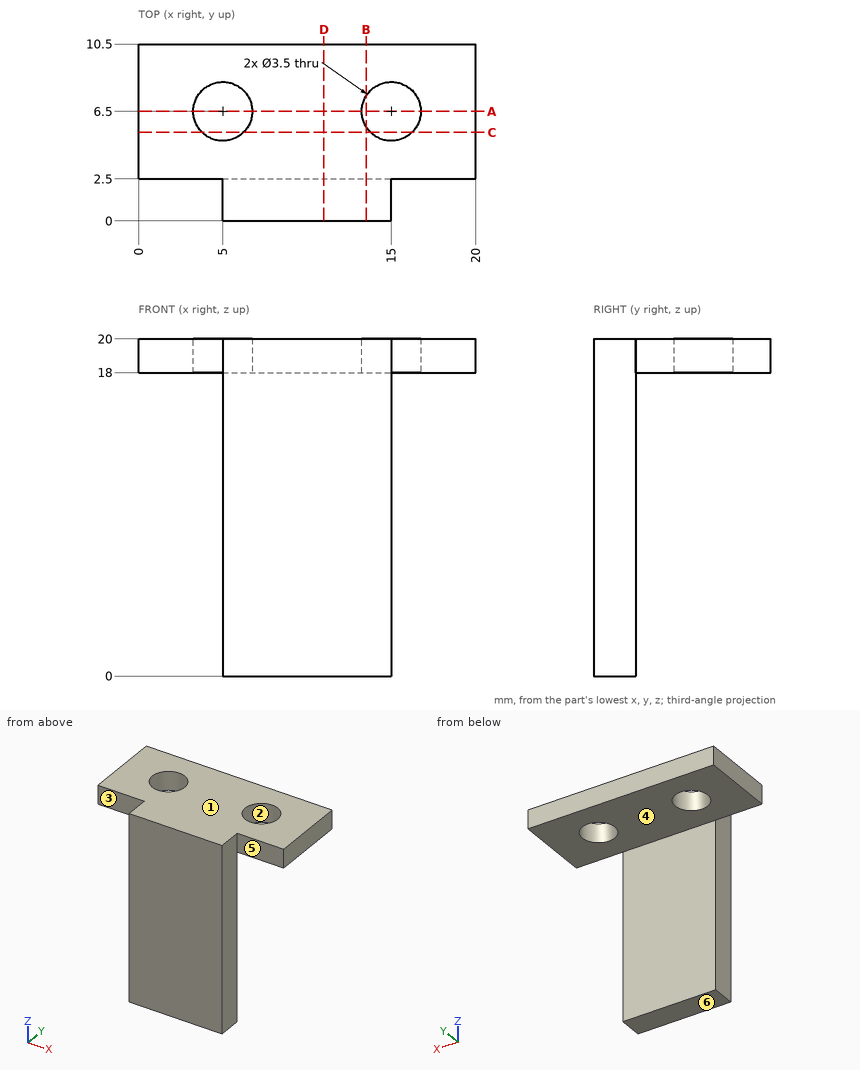
Drawing for the job (mm, zero at the part's lowest x, y, z). A direction names the side the tool comes from. Round coordinates to 2 decimals unless told otherwise and drop trailing zeros. Loops run counter-clockwise (first coordinate to the right, second up) from the corner with the lowest first, then second, coordinate; pieces in that order, holes last. Notation, with made-up numbers: (56.25, 60.25) - (115.25, 60.25) arc R13 ccw to (115.25, 71.25) - close; hole circle Ø6 at (87, 6). An arc over 180 degrees is marked (long way). Write each question's results on one line, items separated by ' | '.
(1) Pin check, flat tips, straight feed: pin 1 (0.6 mm diameter, centred on x = 3, z = 19.5, fed in from -Y); pin 2 (3 mm diameter, centred on y = 1, z = 13, fed in from -X); pin 3 (3 mm diameter, centred on y = 2, z = 9.5, fed in from +X). Stop position of each tip, or through.
Answer below:
pin 1: stops at y = 2.5 | pin 2: stops at x = 5 | pin 3: stops at x = 15
(2) 3-axis set-ups, long thin cutter, end or side, ignore diameter. For the marked faces 3, 4, 5 and 6: which of +Z, -Z, +X, -X, +Y, -Y reach the whole face in a straight line?
Answer below:
face 3: +Z, -Z, -X, -Y | face 4: -Z, +X, -X, +Y | face 5: +Z, -Z, +X, -Y | face 6: -Z, +X, -X, +Y, -Y
(3) Mould opens along X. For the marked faces 1 and 2 say: released by +X, released by -X, zero draft, split by the parting line, or undercut.
Answer below:
face 1: zero draft | face 2: undercut
(4) Saw through at A-A, the plane y = 6.5. List the corners of the cut face in (x, z).
Answer below:
outline: (0, 18) - (3.25, 18) - (3.25, 20) - (0, 20) - close; (6.75, 18) - (13.25, 18) - (13.25, 20) - (6.75, 20) - close; (16.75, 18) - (20, 18) - (20, 20) - (16.75, 20) - close
(5) Saw through at C-C, the plane y = 5.25. List the corners of the cut face in (x, z).
Answer below:
outline: (0, 18) - (3.78, 18) - (3.78, 20) - (0, 20) - close; (6.22, 18) - (13.78, 18) - (13.78, 20) - (6.22, 20) - close; (16.22, 18) - (20, 18) - (20, 20) - (16.22, 20) - close
(6) Saw through at B-B, the plane x = 13.5. List the corners of the cut face in (y, z).
Answer below:
outline: (0, 0) - (2.5, 0) - (2.5, 18) - (5.6, 18) - (5.6, 20) - (0, 20) - close; (7.4, 18) - (10.5, 18) - (10.5, 20) - (7.4, 20) - close
(7) Wall check: L1, parallel to Z at x = 3.25, y = 7; L2, parallel to Y at x = 6.5, z = 7.5; L3, parallel to Y at x = 5.75, z = 18.25. Give the ranges that are in metal, low to high.
Answer below:
L1: z = 18 to 20 | L2: y = 0 to 2.5 | L3: y = 0 to 4.92, 8.08 to 10.5
(8) Saw through at D-D, the plane x = 11. List the corners of the cut face in (y, z).
Answer below:
outline: (0, 0) - (2.5, 0) - (2.5, 18) - (10.5, 18) - (10.5, 20) - (0, 20) - close
